from build123d import *

# Parameters (mm, degrees)
F0_R     = 32.5
F0_R_2   = 27.5
F1_DEPTH = 10
F2_DEPTH = 8.5
F3_DEPTH = 13
F4_R     = 1.5


with BuildPart() as f1:
    # F0 (on Top) → F1 (new body)
    with BuildSketch(Plane.XY):
        Circle(F0_R)
        Circle(F0_R_2, mode=Mode.SUBTRACT)
        Circle(F0_R_2)
        Polygon((-8.55, 4.9363448016), (0, 9.8726896031), (8.55, 4.9363448016), (8.55, -4.9363448016), (0, -9.8726896031), (-8.55, -4.9363448016), align=None, mode=Mode.SUBTRACT)
        Polygon((8.55, 4.9363448016), (0, 9.8726896031), (-8.55, 4.9363448016), (-8.55, -4.9363448016), (0, -9.8726896031), (8.55, -4.9363448016), align=None)
    extrude(amount=F1_DEPTH)

    # F0 (on Top) → F2 (cut)
    with BuildSketch(Plane.XY):
        Polygon((8.55, 4.9363448016), (0, 9.8726896031), (-8.55, 4.9363448016), (-8.55, -4.9363448016), (0, -9.8726896031), (8.55, -4.9363448016), align=None)
    extrude(amount=F2_DEPTH, mode=Mode.SUBTRACT)

    # F0 (on Top) → F3 (join)
    with BuildSketch(Plane.XY):
        Circle(F0_R)
        Circle(F0_R_2, mode=Mode.SUBTRACT)
    extrude(amount=F3_DEPTH)

    # F4
    f4_edges = [f1.edges().sort_by_distance(p)[0] for p in [
        (-32.5, 0, 13),
        (-27.5, 0, 13),
    ]]
    fillet(f4_edges, radius=F4_R)


solid = f1.part
Work out the finished part from the listing and answer in its coordinate system (mm). A direction names the side the tool comes from. Round coordinates to 2 decimals unless told otherwise and drop trailing zeros. Order: outer loops, then holes, each group sorted by start corner. A loop starts at its lowest first (then second) coordinate and runs counter-clockwise, first axis right, second up. Notation, with made-up numbers: M 40.25,75.5 L 58.25,75.5 A14 ccw 58.25,99.5 Z; hole C 75,10.25 d7. An arc over 180 degrees is marked long. One line per item, written item: value.
Q1. For faces 4 (the face through (7, -7, 0)), 5 (the face through (-5.961, -26.846, 10.74)), 6 (the face through (-8.55, 0, 4)), determine the directions among +Z, -Z, +X, -X, +Y, -Y from which every point of the face is accessible in a straight line to the end or side of a thin tool.
Derived:
face 4: -Z, +X, -X, +Y, -Y
face 5: +Z
face 6: -Z
Q2. Find section A-A on y = 0. Write down the section's boundary in (x, z).
Derived:
outline: M -32.5,0 L -8.55,0 L -8.55,8.5 L 8.55,8.5 L 8.55,0 L 32.5,0 L 32.5,11.5 A1.5 ccw 31,13 L 29,13 A1.5 ccw 27.5,11.5 L 27.5,10 L -27.5,10 L -27.5,11.5 A1.5 ccw -29,13 L -31,13 A1.5 ccw -32.5,11.5 Z
Q3. Flat-ended cylindrical pins translate along their axes: pin 1 (4 mm diameter, centred on y = -19, z = 3, fed in from +X); pin 2 (1.5 mm diameter, centred on x = -23, y = 2, fed in from +Z); pin 3 (3 mm diameter, centred on y = -14, z = 5, fed in from +X). Find the tip coordinate at first contact, or state that the pin passes through.
Derived:
pin 1: x = 27.7
pin 2: z = 10
pin 3: x = 30
Q4. Straight lines are drawn through the part: line 1 (Y direction, x = 0, z = 10.75); line 2 (Z direction, x = -1.5, y = 20); line 3 (Y direction, x = 8, z = 3.25). For each, find the intervals that lie inside material, in ascending order.
Derived:
line 1: -32.5 to -27.5, 27.5 to 32.5
line 2: 0 to 10
line 3: -31.5 to -5.25, 5.25 to 31.5
Q5. Determine the mould class of faces 1 (the face through (0, 0, 10)), 2 (the face through (31, 9.76, 5.67)), 3 (the face through (21, -21, 13)) for opening direction X: released by +X, released by -X, zero draft, split by the parting line, or undercut.
Derived:
face 1: undercut
face 2: split by the parting line
face 3: zero draft
Q6. Find section B-B on z = 7.5. Write down the section's boundary in (x, y).
Derived:
outline: C 0,0 d65; hole M -8.55,-4.94 L 0,-9.87 L 8.55,-4.94 L 8.55,4.94 L 0,9.87 L -8.55,4.94 Z
